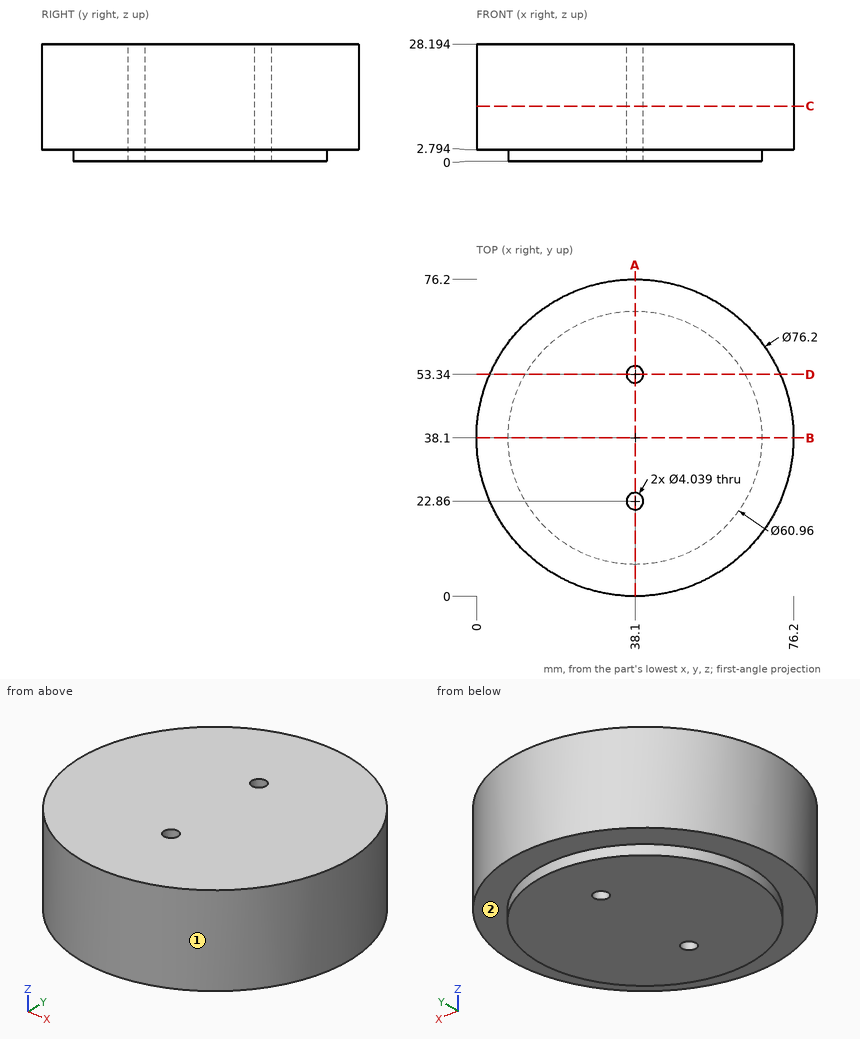
Geometry check sheet. Reference: drawing and pictorial views, mm from the part's lowest x, y, z. Give positions to 0.01 mm unless a question says otherwise; leave off trailing zeros. Write each loop counter-clockwise with the first axis right and the second up, starting at its lowest first coordinate (ties: lowest second). Pieces come first, ordered by that corner, then holes. Notation, with made-up numbers: M 9,81.25 L 52,81.25 A30 ccw 52,109.25 Z; hole C -4.5,-36.75 d6. An arc over 180 degrees is marked long. Use CSV: the item, a comma, the result in double quotes.
1) Material ranges on line 1 along Z through (x, y) = (63, 64); line 2 along Y through (x, z) = (46, 6.25); line 3 along Y through (x, z) = (6, 26) (1 decimal), recorded low to high.
Final values:
line 1,"2.79 to 28.19"
line 2,"0.83 to 75.37"
line 3,"17.6 to 58.6"
2) Go/stop test with flat-tipped pins: pin 1 Ø1 at (y, z) = (12, 19.5) entering from +X; pin 2 Ø10 at (y, z) = (33, 20) entering from +X; pin 3 Ø4 at (y, z) = (31.5, 3.5) entering from +X. Record where each tip stops, or that it passes through.
Final values:
pin 1,"x = 66.32"
pin 2,"x = 76.2"
pin 3,"x = 75.92"
3) Release check for a two-part mould opening along X. For the marked faces 1 and 2 record: released by +X, released by -X, zero draft, split by the parting line, or undercut.
Final values:
face 1,"split by the parting line"
face 2,"zero draft"
4) Cross-section at B-B (y = 38.1). Enter the section's corners in (x, z).
Final values:
outline,"M 0,2.79 L 7.62,2.79 L 7.62,0 L 68.58,0 L 68.58,2.79 L 76.2,2.79 L 76.2,28.19 L 0,28.19 Z"
5) Cross-section at D-D (y = 53.34). Enter the section's corners in (x, z), plus the area to 3 significant figures.
Final values:
outline,"M 3.18,2.79 L 11.7,2.79 L 11.7,0 L 36.08,0 L 36.08,28.19 L 3.18,28.19 Z; M 40.12,0 L 64.5,0 L 64.5,2.79 L 73.02,2.79 L 73.02,28.19 L 40.12,28.19 Z"
area,"1,810 mm²"
6) Cross-section at A-A (x = 38.1). Enter the section's corners in (y, z).
Final values:
outline,"M 0,2.79 L 7.62,2.79 L 7.62,0 L 20.84,0 L 20.84,28.19 L 0,28.19 Z; M 24.88,0 L 51.32,0 L 51.32,28.19 L 24.88,28.19 Z; M 55.36,0 L 68.58,0 L 68.58,2.79 L 76.2,2.79 L 76.2,28.19 L 55.36,28.19 Z"
7) Cross-section at C-C (z = 13.25). Enter the section's corners in (x, y).
Final values:
outline,"C 38.1,38.1 d76.2; hole C 38.1,22.86 d4.04; hole C 38.1,53.34 d4.04"
